The drawing under review shows one solid part. Ordinate dimensions are in mm from its lowest x, y, z. Round coordinates to 2 decimals unless told otherwise and drop trailing zeros. Order: outer loops, then holes, each group sorted by start corner. A loop starts at its lowest first (then second) coordinate and runs counter-clockwise, first axis right, second up. Notation, with made-up numbers: (66, 77.25) - (94, 77.25) arc R28 ccw to (94, 112.25) - close; hole circle Ø4 at (-13.5, 65.5). An arc over 180 degrees is marked (long way). Answer as a JSON object with one key per item and string values. Group by question number.
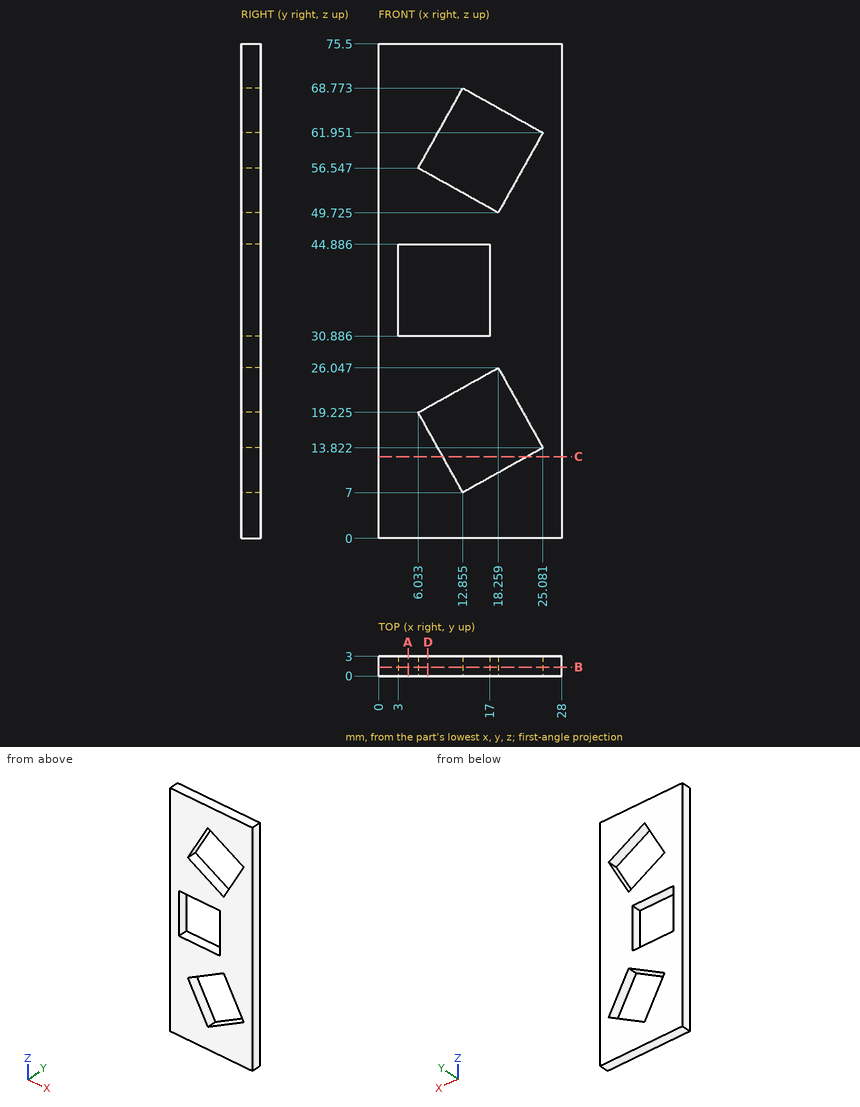
1. Take a section at B-B, the plane y = 1.35. Count the separate pieces of the cut face and the enclosed holes in it, then the cut area to 3 significant figures.
2. To check wall thickness, follow line 1 (Z direction, x = 14, y = 2.5) (1 decimal); line 2 (Z direction, x = 23.5, y = 2.85) (1 decimal); line 3 (Z direction, x = 21.25, y = 2.3) (1 decimal). State the ranges of each line that lie inside material, in increasing order. Write a range as from..to.
3. Take a section at C-C, the plane z = 12.5. Give the boundary of the cut face in (x, y).
4. Clearance check with a flat-ended pin moving along its axis: P1, Ø5, axis at x = 23, z = 40, coming from the -Y side. State where the tip first meets the part, or that it passes through.
5. Take a section at A-A, the plane x = 4.5. Give the boundary of the cut face in (y, z).
6. Take a section at D-D, the plane x = 7.5. Give the boundary of the cut face in (y, z) (1 decimal), then the cut area to 3 significant figures.
Response values:
{
 "1": {"separate pieces": "1", "enclosed holes": "3", "area": "1,530 mm2"},
 "2": {"line 1": "0..7.6, 23.7..30.9, 44.9..52.1, 68.1..75.5", "line 2": "0..12.9, 16.7..59.1, 62.8..75.5", "line 3": "0..11.7, 20.7..55.1, 64.1..75.5"},
 "3": {"outline": "(0, 0) - (9.79, 0) - (9.79, 3) - (0, 3) - close; (22.71, 0) - (28, 0) - (28, 3) - (22.71, 3) - close"},
 "4": {"P1": "y = 0"},
 "5": {"outline": "(0, 0) - (3, 0) - (3, 30.89) - (0, 30.89) - close; (0, 44.89) - (3, 44.89) - (3, 75.5) - (0, 75.5) - close"},
 "6": {"outline": "(0, 0) - (3, 0) - (3, 16.6) - (0, 16.6) - close; (0, 20) - (3, 20) - (3, 30.9) - (0, 30.9) - close; (0, 44.9) - (3, 44.9) - (3, 55.7) - (0, 55.7) - close; (0, 59.2) - (3, 59.2) - (3, 75.5) - (0, 75.5) - close", "area": "164 mm2"}
}
